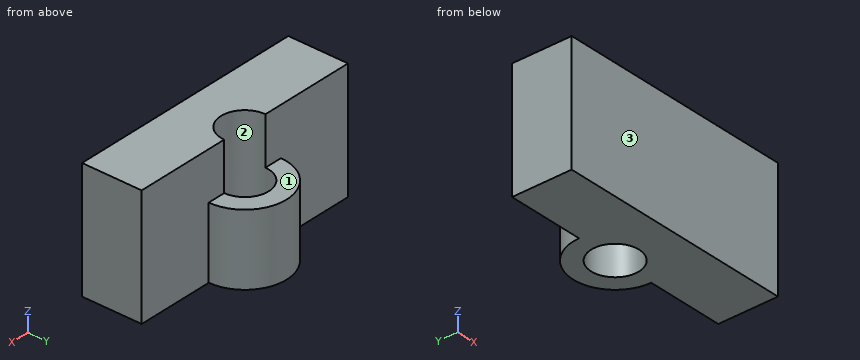
from build123d import *

# Parameters (mm, degrees)
BOSS_EXTRUDE1_DEPTH = 50
BOSS_EXTRUDE2_DEPTH = 30


with BuildPart() as part:
    # Sketch1 → Boss-Extrude1 (new body)
    with BuildSketch(Plane.XY):
        with BuildLine():
            Line((0, 25), (0, 0))
            Line((0, 0), (100, 0))
            Line((100, 0), (100, 25))
            Line((100, 25), (60, 25))
            ThreePointArc((60, 25), (50, 15), (40, 25))
            Line((40, 25), (0, 25))
        make_face()
    extrude(amount=BOSS_EXTRUDE1_DEPTH)

    # Sketch1_3 → Boss-Extrude2 (add)
    with BuildSketch(Plane.XY):
        with BuildLine():
            ThreePointArc((67.5, 25), (50, 42.5), (32.5, 25))
            Line((32.5, 25), (40, 25))
            ThreePointArc((40, 25), (50, 35), (60, 25))
            Line((60, 25), (67.5, 25))
        make_face()
        with BuildLine():
            Line((40, 25), (32.5, 25))
            ThreePointArc((32.5, 25), (50, 7.5), (67.5, 25))
            Line((67.5, 25), (60, 25))
            ThreePointArc((60, 25), (50, 15), (40, 25))
        make_face()
    extrude(amount=BOSS_EXTRUDE2_DEPTH)


solid = part.part
The listing builds one solid part. Answer for the finished solid, in the listing's coordinates (mm). Face numbers are marked on the shaded views. Give positions to 0.01 mm unless a question says otherwise; leave off trailing zeros. Loops run counter-clockwise (first coordinate to the right, second up) from the corner with the lowest first, then second, coordinate; pieces in that order, holes last.
Item 1: A cutting plane is placed at A-A (x = 50). Give the vertices of the cut face in (y, z).
Derived:
outline: (0, 0) - (15, 0) - (15, 50) - (0, 50) - close; (35, 0) - (42.5, 0) - (42.5, 30) - (35, 30) - close
Item 2: A cutting plane is placed at B-B (z = 9). Give the vertices of the cut face in (x, y).
Derived:
outline: (0, 0) - (100, 0) - (100, 25) - (67.5, 25) arc R17.5 ccw to (32.5, 25) - (0, 25) - close; hole circle Ø20 at (50, 25)
Item 3: Determine the mould class of the marked faces 1, 2 and 3 for opening direction Y: +Y half, -Y half, draft (parallel to the pull), parting line (faces both ways), or undercut.
Derived:
face 1: draft
face 2: undercut
face 3: -Y half
Item 4: Find the intervals of material crossed by line 1 along Y through (x, z) = (50, 24.5); line 2 along Z through (x, y) = (66, 31); line 3 along Y through (x, z) = (84, 20), in increasing order.
Derived:
line 1: y = 0 to 15, 35 to 42.5
line 2: z = 0 to 30
line 3: y = 0 to 25
Item 5: Each of these flat-tipped pins is pushed along its axis until it touches: pin 1 Ø1.5 at (x, z) = (50.5, 31.5) entering from +Y; pin 2 Ø5 at (y, z) = (28.5, 27.5) entering from -X; pin 3 Ø8 at (y, z) = (31.5, 17.5) entering from -X; pin 4 Ø16 at (x, y) = (50, 25) entering from +Z. Where does it stop, or does it pass through?
Derived:
pin 1: stops at y = 15.08
pin 2: stops at x = 32.53
pin 3: stops at x = 32.68
pin 4: passes through
Item 6: A cutting plane is placed at D-D (z = 45). Give the vertices of the cut face in (x, y), then the cut area to 3 significant figures.
Derived:
outline: (0, 0) - (100, 0) - (100, 25) - (60, 25) arc R10 cw to (40, 25) - (0, 25) - close
area: 2,340 mm2
Item 7: A cutting plane is placed at C-C (y = 18.5). Give the vertices of the cut face in (x, z).
Derived:
outline: (0, 0) - (42.4, 0) - (42.4, 50) - (0, 50) - close; (57.6, 0) - (100, 0) - (100, 50) - (57.6, 50) - close
